from build123d import *

# Parameters (mm, degrees)
SKETCH1_R           = 1.5
SKETCH1_R_2         = 2
BOSS_EXTRUDE1_DEPTH = 3.175
SKETCH2_R           = 1.5
CUT_EXTRUDE1_DEPTH  = 10
SKETCH3_W           = 264
SKETCH3_H           = 13.5
CUT_EXTRUDE2_DEPTH  = 10
SKETCH4_W           = 264
SKETCH4_H           = 2
CUT_EXTRUDE3_DEPTH  = 10


with BuildPart() as part:
    # Sketch1 → Boss-Extrude1 (new body)
    with BuildSketch(Plane(origin=(0, 0, 0), x_dir=(1, 0, 0), z_dir=(0, 1, 0))):
        Polygon((0, -1.464365857), (264, -1.464365857), (264, 4.535634143), (264, 25.535634143), (0, 25.535634143), align=None)
        with Locations(Location((4, 4.535634143, 0), (0, 0, 270))):
            Circle(SKETCH1_R, mode=Mode.SUBTRACT)
        with Locations(Location((36, 4.535634143, 0), (0, 0, 270))):
            Circle(SKETCH1_R, mode=Mode.SUBTRACT)
        with Locations(Location((228, 4.535634143, 0), (0, 0, 270))):
            Circle(SKETCH1_R, mode=Mode.SUBTRACT)
        with Locations(Location((260, 4.535634143, 0), (0, 0, 270))):
            Circle(SKETCH1_R, mode=Mode.SUBTRACT)
        with Locations(Location((68, 21.535634143, 0), (0, 0, 270))):
            Circle(SKETCH1_R_2, mode=Mode.SUBTRACT)
        with Locations(Location((100, 21.535634143, 0), (0, 0, 270))):
            Circle(SKETCH1_R_2, mode=Mode.SUBTRACT)
        with Locations(Location((132, 21.535634143, 0), (0, 0, 270))):
            Circle(SKETCH1_R_2, mode=Mode.SUBTRACT)
        with Locations(Location((164, 21.535634143, 0), (0, 0, 270))):
            Circle(SKETCH1_R_2, mode=Mode.SUBTRACT)
        with Locations(Location((196, 21.535634143, 0), (0, 0, 270))):
            Circle(SKETCH1_R_2, mode=Mode.SUBTRACT)
    extrude(amount=BOSS_EXTRUDE1_DEPTH)

    # Sketch2 → Cut-Extrude1 (cut)
    with BuildSketch(Plane(origin=(0, 3.175, 0), x_dir=(1, 0, 0), z_dir=(0, 1, 0))):
        with Locations(Location((116, 4.535634143, 0), (0, 0, 270))):
            Circle(SKETCH2_R)
        with Locations(Location((148, 4.535634143, 0), (0, 0, 270))):
            Circle(SKETCH2_R)
        with Locations(Location((100, 4.535634143, 0), (0, 0, 270))):
            Circle(SKETCH2_R)
        with Locations(Location((164, 4.535634143, 0), (0, 0, 270))):
            Circle(SKETCH2_R)
    extrude(amount=-CUT_EXTRUDE1_DEPTH, mode=Mode.SUBTRACT)

    # Sketch3 → Cut-Extrude2 (cut)
    with BuildSketch(Plane(origin=(0, 3.175, 0), x_dir=(1, 0, 0), z_dir=(0, 1, 0))):
        with Locations((132, 18.785634143)):
            Rectangle(SKETCH3_W, SKETCH3_H)
    extrude(amount=-CUT_EXTRUDE2_DEPTH, mode=Mode.SUBTRACT)

    # Sketch4 → Cut-Extrude3 (cut)
    with BuildSketch(Plane(origin=(0, 3.175, 0), x_dir=(1, 0, 0), z_dir=(0, 1, 0))):
        with Locations((132, 11.035634143)):
            Rectangle(SKETCH4_W, SKETCH4_H)
    extrude(amount=-CUT_EXTRUDE3_DEPTH, mode=Mode.SUBTRACT)


solid = part.part
Geometry: final body of the model. Coordinates: model frame, mm. Give positions to 0.01 mm unless a question says otherwise; leave off trailing zeros. Use CSV: the item, a comma, the result in double quotes.
1. Contact query for a flat-ended pin moving along its axis: pin 1 (5 mm diameter, centred on x = 100, z = -4.54, fed in from -Y). Output: stop coordinate, or through.
Answers below:
pin 1,"y = 0"
2. Section query A-A (y = 2.55). Give the number of separate pieces and of enclosed holes in the cut face, plus the area to 3 significant figures.
Answers below:
separate pieces,"1"
enclosed holes,"8"
area,"2,980 mm2"
3. Material intervals for line 1 along Z through (x, y) = (116, 2.5), sorted ascending. Write a range as from..to.
Answers below:
line 1,"-10.04..-6.04, -3.04..1.46"
